Source: CAD feature listing. Evaluate the final solid. Frame: model axes, mm. A direction names the side the tool comes from. Round coordinates to 2 decimals unless told otherwise and drop trailing zeros. Order: outer loops, then holes, each group sorted by start corner. A loop starts at its lowest first (then second) coordinate and runs counter-clockwise, first axis right, second up.
```python
from build123d import *

# Parameters (mm, degrees)
SKETCH1_R           = 56
SKETCH1_R_2         = 2.75
BOSS_EXTRUDE1_DEPTH = 12.5
SKETCH2_R           = 59.175
SKETCH2_R_2         = 56
CUT_EXTRUDE1_DEPTH  = 22.86
CUT_EXTRUDE2_START  = -21
CUT_EXTRUDE2_DEPTH  = 21
FILLET1_R           = 5


with BuildPart() as part:
    # Sketch1 → Boss-Extrude1 (new, symmetric)
    with BuildSketch(Plane.XY):
        with BuildLine():
            Line((-55, -60), (55, -60))
            ThreePointArc((55, -60), (58.535533906, -58.535533906), (60, -55))
            Line((60, -55), (60, 55))
            ThreePointArc((60, 55), (58.535533906, 58.535533906), (55, 60))
            Line((55, 60), (-55, 60))
            ThreePointArc((-55, 60), (-58.535533906, 58.535533906), (-60, 55))
            Line((-60, 55), (-60, -55))
            ThreePointArc((-60, -55), (-58.535533906, -58.535533906), (-55, -60))
        make_face()
        Circle(SKETCH1_R, mode=Mode.SUBTRACT)
        with Locations((-52.5, 52.5)):
            Circle(SKETCH1_R_2, mode=Mode.SUBTRACT)
        with Locations((52.5, 52.5)):
            Circle(SKETCH1_R_2, mode=Mode.SUBTRACT)
        with Locations((52.5, -52.5)):
            Circle(SKETCH1_R_2, mode=Mode.SUBTRACT)
        with Locations((-52.5, -52.5)):
            Circle(SKETCH1_R_2, mode=Mode.SUBTRACT)
    extrude(amount=BOSS_EXTRUDE1_DEPTH, both=True)

    # Sketch2 → Cut-Extrude1 (cut)
    with BuildSketch(Plane(origin=(0, 0, -12.5), x_dir=(-1, 0, 0), z_dir=(0, 0, -1))):
        Circle(SKETCH2_R)
        Circle(SKETCH2_R_2, mode=Mode.SUBTRACT)
    extrude(amount=-CUT_EXTRUDE1_DEPTH, mode=Mode.SUBTRACT)

    # Sketch3 → Cut-Extrude2 (cut)
    with BuildSketch(Plane(origin=(0, 0, -12.5), x_dir=(-1, 0, 0), z_dir=(0, 0, -1)).offset(CUT_EXTRUDE2_START)):
        with BuildLine():
            Line((-60, -22.769071676), (-60, -55))
            ThreePointArc((-60, -55), (-58.535533906, -58.535533906), (-55, -60))
            Line((-55, -60), (-22.769071676, -60))
            ThreePointArc((-22.769071676, -60), (-45.378577683, -45.378577683), (-60, -22.769071676))
        make_face()
        with BuildLine():
            Line((-22.769071676, 60), (-55, 60))
            ThreePointArc((-55, 60), (-58.535533906, 58.535533906), (-60, 55))
            Line((-60, 55), (-60, 22.769071676))
            ThreePointArc((-60, 22.769071676), (-45.378577683, 45.378577683), (-22.769071676, 60))
        make_face()
        with BuildLine():
            Line((60, 22.769071676), (60, 55))
            ThreePointArc((60, 55), (58.535533906, 58.535533906), (55, 60))
            Line((55, 60), (22.769071676, 60))
            ThreePointArc((22.769071676, 60), (45.378577683, 45.378577683), (60, 22.769071676))
        make_face()
        with BuildLine():
            Line((22.769071676, -60), (55, -60))
            ThreePointArc((55, -60), (58.535533906, -58.535533906), (60, -55))
            Line((60, -55), (60, -22.769071676))
            ThreePointArc((60, -22.769071676), (45.378577683, -45.378577683), (22.769071676, -60))
        make_face()
    extrude(amount=CUT_EXTRUDE2_DEPTH, mode=Mode.SUBTRACT)

    # Fillet1
    fillet1_edges = [part.edges().sort_by_distance(p)[0] for p in [
        (-45.378577683, -45.378577683, 8.5),
        (45.378577683, 45.378577683, 8.5),
        (45.378577683, -45.378577683, 8.5),
        (-45.378577683, 45.378577683, 8.5),
    ]]
    fillet(fillet1_edges, radius=FILLET1_R)


solid = part.part
```
1. Pull-direction query (Y, two-part tool) for faces 1 (the face through (-1, -60, 3)), 2 (the face through (-54.527, -50.641, 10.472)), 3 (the face through (51, -50, 8.5)), 4 (the face through (50.473, 54.359, 10.472)); classes: released by +Y, released by -Y, zero draft, split by the parting line, or undercut.
2. Access query for faces 5 (the face through (-50, -54, 8.5)), 6 (the face through (-45.109, 45.646, -4.388)), 7 (the face through (50, 50, 8.5)), 8 (the face through (-58, 59, 11)). Directions: +Z, -Z, +X, -X, +Y, -Y. A direction counts if a zero-diameter tool reaches every point of the face in a straight line with its end or side. Return the directions, or none.
3. First-contact query: pin 1 (4.5 mm diameter, centred on x = -52.5, y = -52.5, fed in from +Z); pin 2 (2 mm diameter, centred on x = 40.5, z = -7, fed in from -Y); pin 3 (12 mm diameter, centred on x = 37, z = -1.5, fed in from -Y); pin 4 (10 mm diameter, centred on y = 28, z = 1, fed in from -X). Flat tips, straight axial feed; report the tip coordinate or a pass-through.
4. Section C-C on x = 7. Return loops of the section in (y, z).
5. Section B-B on z = -10.5. Return loops of the section in (x, y) (3 decimals), plus the area to 3 significant figures.
6. Line query: line 1 along X through (y, z) = (-52.5, 10.1); line 2 along Y through (x, z) = (0, -6.25) (3 decimals); line 3 along Y through (x, z) = (-7.5, 7). Output: solid intervals per line, ascending.
7. Section A-A on y = 0. Return loops of the section in (x, z) (3 decimals).
8. Section D-D on y = 52.5. State how many separate pieces and enclosed holes the cut face has, plus the area to 3 significant figures.
Result:
1. face 1: released by -Y
1. face 2: undercut
1. face 3: zero draft
1. face 4: undercut
2. face 5: -Z, -X, -Y
2. face 6: -Z, -X, +Y
2. face 7: -Z, +X, +Y
2. face 8: +Z, -Z, -X, +Y
3. pin 1: passes through
3. pin 2: stops at y = -50.58
3. pin 3: stops at y = -56.19
3. pin 4: stops at x = -59.91
4. outline: (-60, -12.5) - (-58.76, -12.5) - (-58.76, 10.36) - (-55.56, 10.36) - (-55.56, 12.5) - (-60, 12.5) - close; (55.56, 10.36) - (58.76, 10.36) - (58.76, -12.5) - (60, -12.5) - (60, 12.5) - (55.56, 12.5) - close
5. outline: (-60, -22.769) arc R64.175 ccw to (-22.769, -60) - (22.769, -60) arc R64.175 ccw to (60, -22.769) - (60, 22.769) arc R64.175 ccw to (22.769, 60) - (-22.769, 60) arc R64.175 ccw to (-60, 22.769) - close; hole circle Ø118.35 at (0, 0)
5. area: 1,430 mm2
6. line 1: x = -60 to -55.25, -49.75 to -27.3, 27.3 to 49.75, 55.25 to 60
6. line 2: y = -60 to -59.175, 59.175 to 60
6. line 3: y = -60 to -58.7, 58.7 to 60
7. outline: (-60, -12.5) - (-59.175, -12.5) - (-59.175, 10.36) - (-56, 10.36) - (-56, 12.5) - (-60, 12.5) - close; (56, 10.36) - (59.175, 10.36) - (59.175, -12.5) - (60, -12.5) - (60, 12.5) - (56, 12.5) - close
8. separate pieces: 4
8. enclosed holes: 0
8. area: 673 mm2
